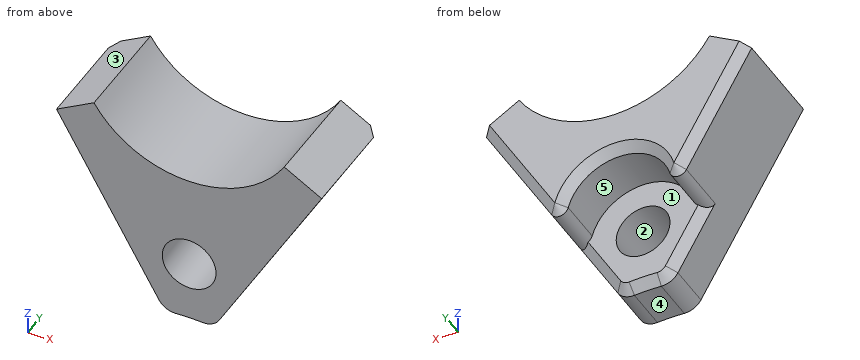
from build123d import *

# Parameters (mm, degrees)
SKETCH1_R                = 1.5
BASE_DEPTH               = 5.9
FASTENER_CLEARANCE_DEPTH = 3
FASTENER_FILLET_R        = 0.5
BASE_FILLET_R            = 1
BODY_CHAMFER_SIZE        = 0.5


with BuildPart() as part:
    # Sketch1 → Base (new body)
    with BuildSketch(Plane(origin=(0, 0, 0), x_dir=(1, 0, 0), z_dir=(0, 1, 0))):
        with BuildLine():
            Line((5.307777313, 3.3), (7.397782409, 4.506665005))
            Line((7.397782409, 4.506665005), (1.360112218, 14.964216534))
            ThreePointArc((1.360112218, 14.964216534), (0, 14.89), (-1.360112218, 14.964216534))
            Line((-1.360112218, 14.964216534), (-7.397782409, 4.506665005))
            Line((-7.397782409, 4.506665005), (-5.307777313, 3.3))
            ThreePointArc((-5.307777313, 3.3), (0, 6.25), (5.307777313, 3.3))
        make_face()
        with Locations((0, 11.5)):
            Circle(SKETCH1_R, mode=Mode.SUBTRACT)
    extrude(amount=BASE_DEPTH)

    # Sketch2 → Fastener Clearance (cut)
    with BuildSketch(Plane(origin=(0, 5.9, 0), x_dir=(1, 0, 0), z_dir=(0, 1, 0))):
        with BuildLine():
            Line((-2.762208294, 12.535714894), (-1.360112218, 14.964216534))
            ThreePointArc((-1.360112218, 14.964216534), (0, 14.89), (1.360112218, 14.964216534))
            Line((1.360112218, 14.964216534), (2.762208294, 12.535714894))
            ThreePointArc((2.762208294, 12.535714894), (0, 8.55), (-2.762208294, 12.535714894))
        make_face()
    extrude(amount=-FASTENER_CLEARANCE_DEPTH, mode=Mode.SUBTRACT)

    # Fastener Fillet
    fastener_fillet_edges = [part.edges().sort_by_distance(p)[0] for p in [
        (2.762208294, 4.4, -12.535714894),
        (-2.762208294, 4.4, -12.535714894),
    ]]
    fillet(fastener_fillet_edges, radius=FASTENER_FILLET_R)

    # Base Fillet
    base_fillet_edges = [part.edges().sort_by_distance(p)[0] for p in [
        (-1.360112218, 1.45, -14.964216534),
        (1.360112218, 1.45, -14.964216534),
    ]]
    fillet(base_fillet_edges, radius=BASE_FILLET_R)

    # Body Chamfer
    body_chamfer_edges = [part.edges().sort_by_distance(p)[0] for p in [
        (5.576129132, 5.9, -7.661861034),
        (2.219874831, 2.9, -13.475064006),
        (0, 5.9, -8.55),
        (-5.576129132, 5.9, -7.661861034),
        (-3.259182505, 5.9, -11.063163021),
        (3.259182505, 5.9, -11.063163021),
        (-2.219874831, 2.9, -13.475064006),
        (0, 2.9, -14.89),
        (1.285248704, 2.9, -14.795081779),
        (-1.285248704, 2.9, -14.795081779),
    ]]
    chamfer(body_chamfer_edges, length=BODY_CHAMFER_SIZE)


solid = part.part
Here's how the part is built. I have some questions about the finished solid (model axes, mm). Face numbers are marked on the shaded views. A direction names the side the tool comes from. Round coordinates to 2 decimals unless told otherwise and drop trailing zeros. Write each loop counter-clockwise with the first axis right and the second up, starting at its lowest first coordinate (ties: lowest second). Pieces come first, ordered by that corner, then holes.
1. I need wall thicknesses on L1, parallel to Z at x = 0, y = 1.3; L2, parallel to X at y = 1.75, z = -4.75; L3, parallel to Y at x = -0.25, z = -14. Which ranges of each line are inside material? Lowest first, please.
2. Will these pins go through, and if not, where does the flat tip stop? pin 1 Ø2 at (x, y) = (4, 5) entering from +Z; pin 2 Ø2 at (x, y) = (5.5, 2) entering from +Z.
3. Suppose I cut it at C-C (z = -11.5). List the corners of the cut face in (x, y) for me, and give its area (3 significant figures).
4. Suppose I cut it at D-D (y = 3.95). List the corners of the cut face in (x, z) for me, and give its area (3 significant figures).
5. If we mould it in two halves opening along Z, with no side actions, what happens to the marked faces 1, 2 and 3? For each: released by +Z, released by -Z, zero draft, split by the parting line, or undercut.
6. Suppose I cut it at B-B (x = 0). List the corners of the cut face in (y, z) for me.
7. For the marked faces 4 and 5, which set-ups out of +Z, -Z, +X, -X, +Y, -Y let a thin tool reach every point of the face, with its end or its side?
8. Suppose I cut it at A-A (y = 1.7). List the corners of the cut face in (x, z) for me, and give its area (3 significant figures).
Answer sheet:
1. L1: z = -14.89 to -13, -10 to -6.25
1. L2: x = -7.26 to -4.06, 4.06 to 7.26
1. L3: y = 0 to 2.9
2. pin 1: stops at z = -3.75
2. pin 2: stops at z = -3.3
3. outline: (-3.36, 0) - (-1.5, 0) - (-1.5, 2.9) - (-2.78, 2.9) - (-3.36, 2.4) - close; (1.5, 0) - (3.36, 0) - (3.36, 2.4) - (2.78, 2.9) - (1.5, 2.9) - close
3. area: 10.5 mm2
4. outline: (-7.4, -4.51) - (-3.75, -10.82) arc R0.5 ccw to (-2.84, -10.7) arc R2.95 cw to (2.84, -10.7) arc R0.5 ccw to (3.75, -10.82) - (7.4, -4.51) - (5.31, -3.3) arc R6.25 cw to (-5.31, -3.3) - close
4. area: 54.2 mm2
5. face 1: zero draft
5. face 2: undercut
5. face 3: released by +Z
6. outline: (0, -14.89) - (2.4, -14.89) - (2.9, -14.39) - (2.9, -13) - (0, -13) - close; (0, -10) - (2.9, -10) - (2.9, -8.55) - (5.4, -8.55) - (5.9, -8.05) - (5.9, -6.25) - (0, -6.25) - close
7. face 4: -Z, +Y, -Y
7. face 5: -Z, +Y
8. outline: (-7.4, -4.51) - (-1.68, -14.41) arc R1 ccw to (-0.75, -14.91) arc R12.5 cw to (0.75, -14.91) arc R1 ccw to (1.68, -14.41) - (7.4, -4.51) - (5.31, -3.3) arc R6.25 cw to (-5.31, -3.3) - close; hole circle Ø3 at (0, -11.5)
8. area: 77.5 mm2
